The drawing under review shows one solid part. Ordinate dimensions are in mm from its lowest x, y, z. Coordinates: 2 decimals unless noted, no trailing zeros. Write each loop counter-clockwise with the first axis right and the second up, starting at its lowest first coordinate (ties: lowest second). Pieces come first, ordered by that corner, then holes. Notation, with made-up numbers: M -21.75,-6 L 4.25,-6 A36 ccw 4.25,29 Z; hole C 79,-8 d5. An arc over 180 degrees is marked long. Write each question's results on one line, items separated by ' | '. Start each with the question number.
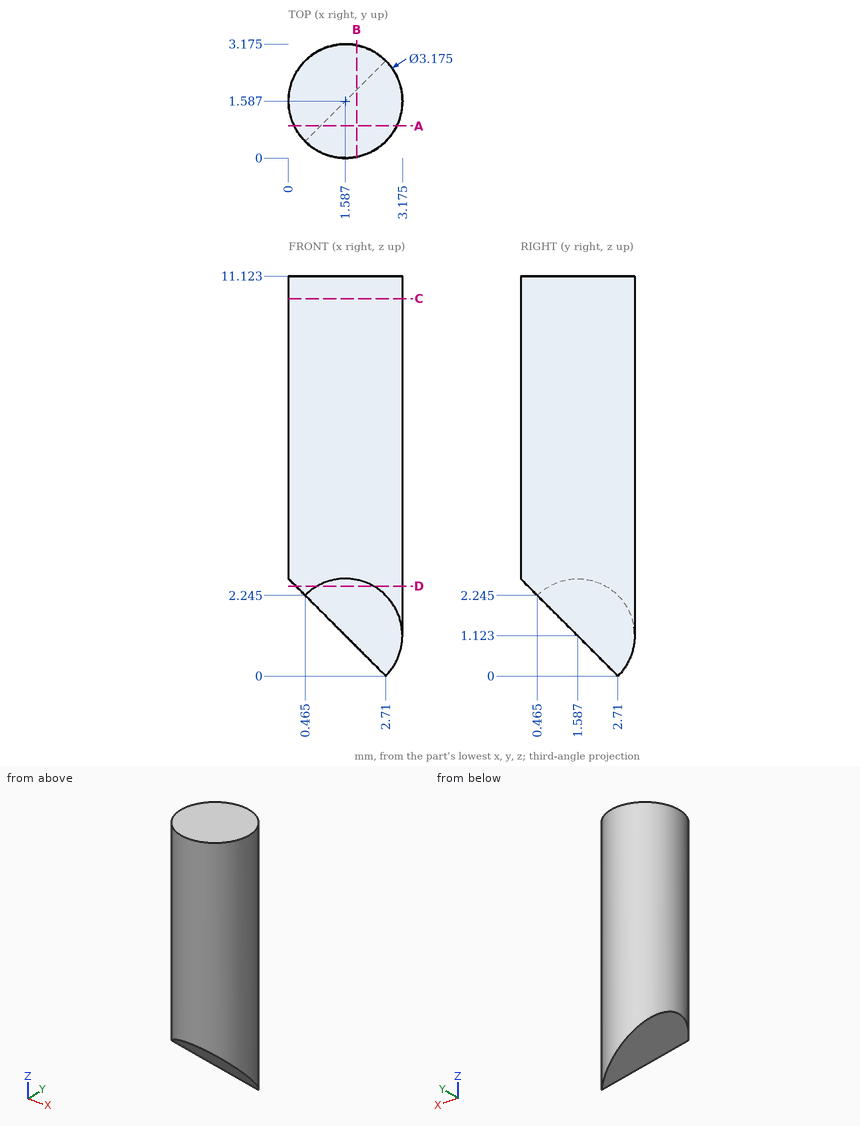
Item 1: We need section C-C on z = 10.5. State the section outline as (x, y) points (1 decimal).
Item 2: We need section B-B on x = 1.9. State the section outline as (y, z) points.
Item 3: We need section A-A on y = 0.9. State the section outline as (x, z) points.
Item 4: We need section D-D on z = 2.5. State the section outline as (x, y) points (1 decimal).
Item 5: Wall thickness on L1, parallel to Z at x = 1.65, y = 0.6 (1 decimal); L2, parallel to Z at x = 2.25, y = 1.75 (1 decimal); L3, parallel to X at y = 2.7, z = 5.5 (1 decimal): over which ranges is each line inside the solid? List them lowest first.
Answer:
1) outline: C 1.6,1.6 d3.2
2) outline: M 0.03,2.68 L 1.9,0.81 L 3.14,0.81 L 3.14,11.12 L 0.03,11.12 Z
3) outline: M 0.16,2.55 L 0.9,1.81 L 3.02,1.81 L 3.02,11.12 L 0.16,11.12 Z
4) outline: M 0.2,0.8 A1.6 ccw 0.8,0.2 L 2.4,0.2 A1.6 ccw long 0.2,2.4 Z
5) L1: z = 2.1 to 11.1 | L2: z = 1 to 11.1 | L3: x = 0.5 to 2.7
